For this review, take the finished solid that the model builds, in its own axes (mm). A direction names the side the tool comes from. Coordinates: 2 decimals unless noted, no trailing zeros. Write each loop counter-clockwise with the first axis right and the second up, starting at its lowest first coordinate (ties: lowest second). Pieces come first, ordered by that corner, then holes. Notation, with made-up numbers: (-36, 82) -> (-8, 82) arc R25 ccw to (-8, 106) -> close; hole circle Ø4 at (79.5, -10). An arc over 180 degrees is marked (long way). One line per item, written item: value. Start each with the question number.
1) Mouldability with a two-part tool opening along X and no side actions: class faces 3 (the cylindrical face through (30.07, -16.99, 24.04)), 4 (the cylindrical face through (-5.598, 42.634, 23.232)), 5 (the cylindrical face through (-0.325, 34.536, 24.044)), 6 (the flat face through (9, 1, 24.5)) as released by +X, released by -X, zero draft, split by the parting line, or undercut.
2) Add section C-C (y = -18). State the section outline as (x, z) points, and give its area (3 significant figures).
3) Machinability: for faces 1 (the cylindrical face through (-32.282, -16.986, 24.044)), 2 (the cylindrical face through (-5.158, 3.955, 19.535)), which of the approach directions +Z, -Z, +X, -X, +Y, -Y give a long, thin tool a straight path to every point of the face, cutting with its end or side? Answer none if there is none.
4) Add section D-D (y = 36). State the section outline as (x, z) points, and give its area (3 significant figures).
5) Add section B-B (y = 0). State the section outline as (x, z) points.
6) For pin 1 Ø3 at (x, z) = (3, 23) entering from -Y; pin 2 Ø4 at (y, z) = (-26.5, 20.5) entering from -X; pin 3 Ø1 at (x, z) = (6, 22.5) entering from -Y, all flat-tipped, find the tip position at first contact; note any pin that passes through.
7) Add section A-A (x = 0). State the section outline as (y, z) points, and give its area (3 significant figures).
8) For probe 1 along Y at (x, z) = (0, 24.1); probe 2 along X at (y, z) = (0, 21.25); probe 3 along Z at (x, y) = (-1, 14.5), list the stretches that pass through material, from the lowest coordinate up. Write a range as from..to.
from build123d import *

# Parameters (mm, degrees)
SKETCH006_R     = 43
SKETCH006_R_2   = 1.5
SKETCH006_R_3   = 4
PAD_DEPTH       = 2.5
CHAMFER001_SIZE = 1.6
SKETCH_R        = 6.5
SKETCH_R_2      = 4
PAD001_DEPTH    = 5
CHAMFER_SIZE    = 1


with BuildPart() as part:
    # Sketch006 → Pad (new body)
    with BuildSketch(Plane.XY.offset(22)):
        Circle(SKETCH006_R)
        with Locations((0, 36)):
            Circle(SKETCH006_R_2, mode=Mode.SUBTRACT)
        with Locations((31.176915, -18)):
            Circle(SKETCH006_R_2, mode=Mode.SUBTRACT)
        with Locations((-31.176915, -18)):
            Circle(SKETCH006_R_2, mode=Mode.SUBTRACT)
        Circle(SKETCH006_R_3, mode=Mode.SUBTRACT)
    extrude(amount=PAD_DEPTH)

    # Chamfer001
    chamfer001_edges = [part.edges().sort_by_distance(p)[0] for p in [
        (-32.676915, -18, 22),
        (29.676915, -18, 22),
        (-1.5, 36, 22),
    ]]
    chamfer(chamfer001_edges, length=CHAMFER001_SIZE)

    # Sketch (on Face4 of Chamfer001) → Pad001 (join)
    with BuildSketch(Plane(origin=(0, 0, 22), x_dir=(1, 0, 0), z_dir=(0, 0, -1))):
        Circle(SKETCH_R)
        Circle(SKETCH_R_2, mode=Mode.SUBTRACT)
    extrude(amount=PAD001_DEPTH)

    # Chamfer
    chamfer_edges = [part.edges().sort_by_distance(p)[0] for p in [
        (-4, 0, 24.5),
    ]]
    chamfer(chamfer_edges, length=CHAMFER_SIZE)


solid = part.part
Numbers:
1. face 3: undercut
1. face 4: split by the parting line
1. face 5: undercut
1. face 6: zero draft
2. outline: (-39.05, 22) -> (-34.28, 22) -> (-32.68, 23.6) -> (-32.68, 24.5) -> (-39.05, 24.5) -> close; (-29.68, 23.6) -> (-28.08, 22) -> (28.08, 22) -> (29.68, 23.6) -> (29.68, 24.5) -> (-29.68, 24.5) -> close; (32.68, 23.6) -> (34.28, 22) -> (39.05, 22) -> (39.05, 24.5) -> (32.68, 24.5) -> close
2. area: 175 mm²
3. face 1: +Z, -Z
3. face 2: -Z
4. outline: (-23.52, 22) -> (-3.1, 22) -> (-1.5, 23.6) -> (-1.5, 24.5) -> (-23.52, 24.5) -> close; (1.5, 23.6) -> (3.1, 22) -> (23.52, 22) -> (23.52, 24.5) -> (1.5, 24.5) -> close
4. area: 108 mm²
5. outline: (-43, 22) -> (-6.5, 22) -> (-6.5, 17) -> (-4, 17) -> (-4, 23.5) -> (-5, 24.5) -> (-43, 24.5) -> close; (4, 17) -> (6.5, 17) -> (6.5, 22) -> (43, 22) -> (43, 24.5) -> (5, 24.5) -> (4, 23.5) -> close
6. pin 1: y = -42.97
6. pin 2: x = -34.86
6. pin 3: y = -42.65
7. outline: (-43, 22) -> (-6.5, 22) -> (-6.5, 17) -> (-4, 17) -> (-4, 23.5) -> (-5, 24.5) -> (-43, 24.5) -> close; (4, 17) -> (6.5, 17) -> (6.5, 22) -> (32.9, 22) -> (34.5, 23.6) -> (34.5, 24.5) -> (5, 24.5) -> (4, 23.5) -> close; (37.5, 23.6) -> (39.1, 22) -> (43, 22) -> (43, 24.5) -> (37.5, 24.5) -> close
7. area: 209 mm²
8. probe 1: -43..-4.6, 4.6..34.5, 37.5..43
8. probe 2: -6.5..-4, 4..6.5
8. probe 3: 22..24.5
